```python
from build123d import *

# Parameters (mm, degrees)
SKETCH1_W           = 44
SKETCH1_H           = 20
BOSS_EXTRUDE1_DEPTH = 7
SKETCH3_R           = 8
BOSS_EXTRUDE2_DEPTH = 13
SKETCH4_R           = 7
CUT_EXTRUDE1_DEPTH  = 2
SKETCH5_W           = 1.5
SKETCH5_H           = 1.5
BOSS_EXTRUDE3_DEPTH = 7


with BuildPart() as part:
    # Sketch1 → Boss-Extrude1 (new body)
    with BuildSketch(Plane(origin=(0, 0, 0), x_dir=(1, 0, 0), z_dir=(0, 1, 0))):
        with Locations((-3.680933852, 5.151750973)):
            Rectangle(SKETCH1_W, SKETCH1_H)
    extrude(amount=BOSS_EXTRUDE1_DEPTH)

    # Sketch3 → Boss-Extrude2 (add)
    with BuildSketch(Plane(origin=(0, 7, 0), x_dir=(1, 0, 0), z_dir=(0, 1, 0))):
        with Locations((-16.180933852, 5.151750973)):
            Circle(SKETCH3_R)
        with Locations((8.819066148, 5.151750973)):
            Circle(SKETCH3_R)
    extrude(amount=BOSS_EXTRUDE2_DEPTH)

    # Sketch4 → Cut-Extrude1 (cut)
    with BuildSketch(Plane(origin=(0, 20, 0), x_dir=(1, 0, 0), z_dir=(0, 1, 0))):
        with Locations((-16.180933852, 5.151750973)):
            Circle(SKETCH4_R)
        with Locations((8.819066148, 5.151750973)):
            Circle(SKETCH4_R)
    extrude(amount=-CUT_EXTRUDE1_DEPTH, mode=Mode.SUBTRACT)

    # Sketch5 → Boss-Extrude3 (add)
    with BuildSketch(Plane.XY.offset(4.848249027)):
        with Locations((-7.930933852, 6.25)):
            Rectangle(SKETCH5_W, SKETCH5_H)
        with Locations((-4.930933852, 6.25)):
            Rectangle(SKETCH5_W, SKETCH5_H)
        with Locations((-1.930933852, 6.25)):
            Rectangle(SKETCH5_W, SKETCH5_H)
        with Locations((1.069066148, 6.25)):
            Rectangle(SKETCH5_W, SKETCH5_H)
    extrude(amount=BOSS_EXTRUDE3_DEPTH)


solid = part.part
```
Input: part model. Units: mm. Frame: model coordinates. A direction names the side the tool comes from. Round coordinates to 2 decimals unless told otherwise and drop trailing zeros. Loops run counter-clockwise (first coordinate to the right, second up) from the corner with the lowest first, then second, coordinate; pieces in that order, holes last. Notation, with made-up numbers: (4.5, -26.75) -> (50.5, -26.75) arc R36 ccw to (50.5, 9.25) -> close; hole circle Ø1 at (31.5, 16.5). An arc over 180 degrees is marked (long way). Write each question's results on one line, items separated by ' | '.
1. Section B-B (x = 4). Return loops of the section in (y, z), and give its area (3 significant figures).
Geometry results:
outline: (0, -15.15) -> (7, -15.15) -> (7, -11.54) -> (20, -11.54) -> (20, -10.23) -> (18, -10.23) -> (18, -0.07) -> (20, -0.07) -> (20, 1.23) -> (7, 1.23) -> (7, 4.85) -> (0, 4.85) -> close | area: 286 mm2
2. First-contact query: P1, Ø1, axis at y = 9.5, z = 3.5, coming from the -X side; P2, Ø1.2, axis at y = 6, z = 9, coming from the -X side; P3, Ø2, axis at x = 13.5, z = -2.5, coming from the +Y side; P4, Ø1.2, axis at y = 6.5, z = 9.5, coming from the +X side. Flat tips, straight axial feed; report the tip coordinate or a pass-through.
Geometry results:
P1: through | P2: x = -8.68 | P3: y = 18 | P4: x = 1.82
3. Set-up query: faces 1 (the face through (-16, 18, -5)), 2 (the face through (-8.681, 6, 8)), 3 (the face through (-4.181, 6, 8)), 4 (the face through (-5, 5.5, 8)). Return all of +Z, -Z, +X, -X, +Y, -Y with unobstructed straight access to the full face (end or side cutting, diameter ignored); none if empty.
Geometry results:
face 1: +Y | face 2: +Z, -X, +Y, -Y | face 3: +Z, +Y, -Y | face 4: +Z, +X, -X, -Y
4. Section C-C (z = 1). Return loops of the section in (x, y).
Geometry results:
outline: (-25.68, 0) -> (18.32, 0) -> (18.32, 7) -> (13.93, 7) -> (13.93, 20) -> (12.16, 20) -> (12.16, 18) -> (5.48, 18) -> (5.48, 20) -> (3.7, 20) -> (3.7, 7) -> (-11.07, 7) -> (-11.07, 20) -> (-12.84, 20) -> (-12.84, 18) -> (-19.52, 18) -> (-19.52, 20) -> (-21.3, 20) -> (-21.3, 7) -> (-25.68, 7) -> close
5. Mould query, pull axis Z, two halves, no side actions, for faces 5 (the face through (7.908, 19.014, -12.092)), 6 (the face through (-2, 6, 11.848)), 7 (the face through (-5.681, 6, 8)). Classes: +Z half, -Z half, draft (parallel to the pull), parting line (faces both ways), or undercut.
Geometry results:
face 5: undercut | face 6: +Z half | face 7: draft
6. Ray query, line 1 (X direction, y = 6.75, z = 6); line 2 (Z direction, x = -22.5, y = 2.5); line 3 (Y direction, x = -5, z = -11.5). Return the intervals inside material, ascending. Write a range as from..to.
Geometry results:
line 1: -8.68..-7.18, -5.68..-4.18, -2.68..-1.18, 0.32..1.82 | line 2: -15.15..4.85 | line 3: 0..7
7. Section D-D (y = 17.25). Return loops of the section in (x, z).
Geometry results:
outline: circle Ø16 at (-16.18, -5.15); circle Ø16 at (8.82, -5.15)
8. Section A-A (z = 8.5). Return loops of the section in (x, y).
Geometry results:
outline: (-8.68, 5.5) -> (-7.18, 5.5) -> (-7.18, 7) -> (-8.68, 7) -> close; (-5.68, 5.5) -> (-4.18, 5.5) -> (-4.18, 7) -> (-5.68, 7) -> close; (-2.68, 5.5) -> (-1.18, 5.5) -> (-1.18, 7) -> (-2.68, 7) -> close; (0.32, 5.5) -> (1.82, 5.5) -> (1.82, 7) -> (0.32, 7) -> close
